For this review, use the dimensioned drawing (mm, ordinates from the lowest corner) and the shaded views. Coordinates: 2 decimals unless noted, no trailing zeros. Loops run counter-clockwise (first coordinate to the right, second up) from the corner with the lowest first, then second, coordinate; pieces in that order, holes last. Notation, with made-up numbers: (60, 70.5) - (66, 70.5) arc R24 ccw to (66, 97.5) - close; hole circle Ø6 at (43.5, 84.5). An arc over 180 degrees is marked (long way). Answer in a Markdown table with one row per item. Add a question column.
(1) We need section A-A, the plane z = 102. Write out the cut boundary in (x, y) (1 decimal).
(2) Clearance check with flat-ended pins moving along their axes: pin 1 (6 mm diameter, centred on x = 4, z = 122, fed in from -Y); pin 2 (2 mm diameter, centred on y = 4.5, z = 53.5, fed in from +X); pin 3 (1 mm diameter, centred on y = 7.5, z = 72, fed in from -X). State where each tip first meets the part, or that it passes through.
(3) To check wall thickness, follow L1, parallel to Y at x = 11, z = 160 (1 decimal); L2, parallel to Y at x = 8, z = 92.5; L3, parallel to X at y = 4.5, z = 154.5. State the ranges of each line that lie inside material, in increasing order. Write a range as [from, to].
(4) We need section B-B, the plane z = 141. Write out the cut boundary in (x, y) (1 decimal).
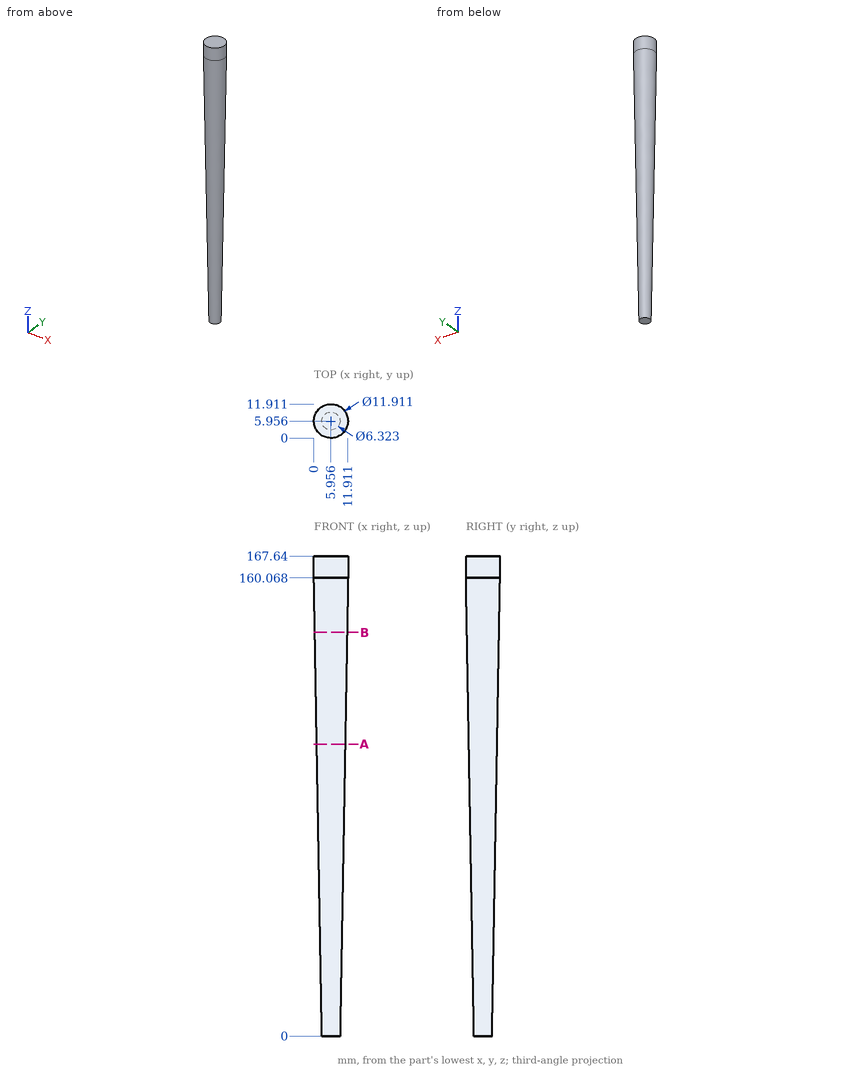
Responses:
| question | item | result |
|---|---|---|
| 1 | outline | circle Ø9.9 at (6, 6) |
| 2 | pin 1 | stops at y = 0.62 |
| 2 | pin 2 | stops at x = 10.03 |
| 2 | pin 3 | stops at x = 1.66 |
| 3 | L1 | y = [2.8, 9.1] |
| 3 | L2 | y = [1.64, 10.27] |
| 3 | L3 | x = [0.28, 11.63] |
| 4 | outline | circle Ø11.2 at (6, 6) |
